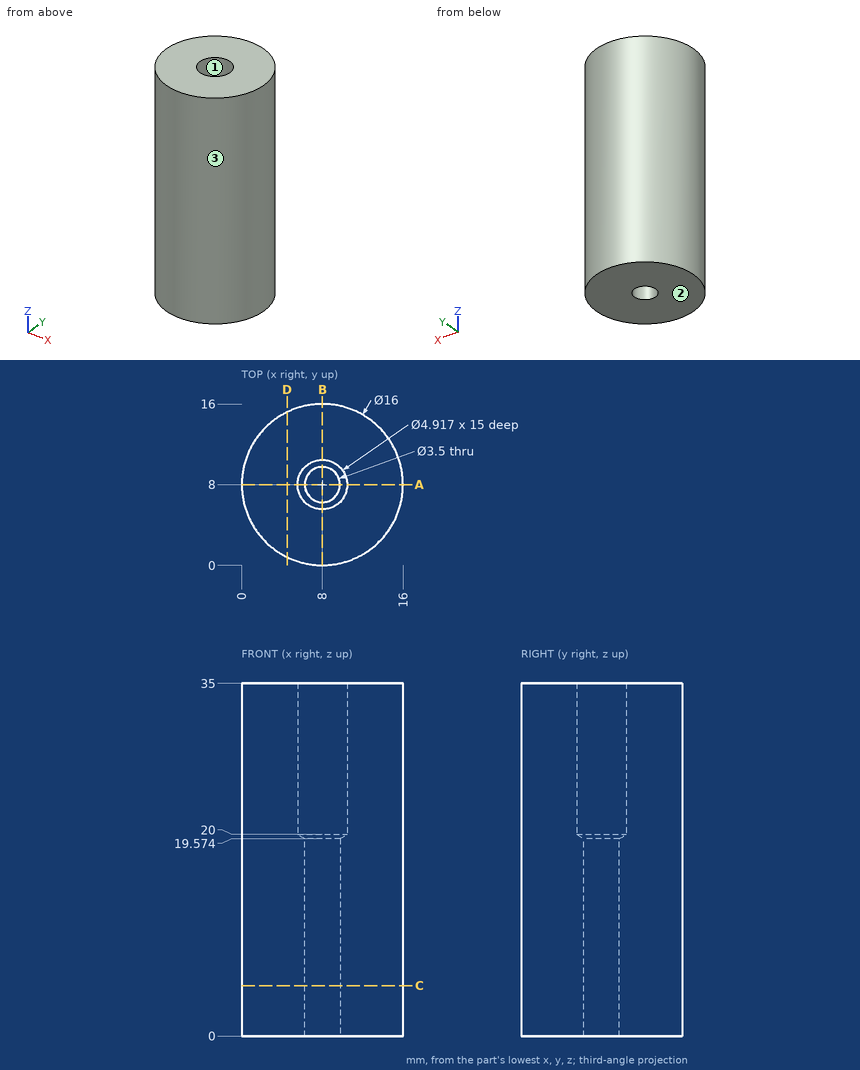
Check sheet for the drawn part. Datum: minimum x, y, z corner. Units: mm. Round coordinates to 2 decimals unless told otherwise and drop trailing zeros. Order: outer loops, then holes, each group sorted by start corner. A loop starts at its lowest first (then second) coordinate and runs counter-clockwise, first axis right, second up. Notation, with made-up numbers: (-24.75, 57) -> (-7.75, 57) arc R18 cw to (-7.75, 90) -> close; hole circle Ø10 at (54, 36). An arc over 180 degrees is marked (long way). Use CSV: the item, a comma, the result in double quotes.
(1) Draft check along Y on the marked faces 1, 2 and 3. Enter one of: pulls with the +Y half, pulls with the -Y half, needs draft (parallel to the pull), parting line crosses it, or undercut.
Worked out:
face 1,"undercut"
face 2,"needs draft"
face 3,"parting line crosses it"
(2) Depth check by flat-ended pin: pin 1 (1.5 mm diameter, centred on y = 4.5, z = 12.5, fed in from +X); pin 2 (2 mm diameter, centred on y = 6.5, z = 29.5, fed in from -X); pin 3 (1 mm diameter, centred on x = 10.5, z = 20.5, fed in from +Y). Enter the tip coordinate at first touch or a pass-through.
Worked out:
pin 1,"x = 15.51"
pin 2,"x = 0.02"
pin 3,"y = 15.75"
(3) Cross-section at C-C (z = 5). Record the boundary of the cut face in (x, y), and give its area (3 significant figures).
Worked out:
outline,"circle Ø16 at (8, 8); hole circle Ø3.5 at (8, 8)"
area,"191 mm²"
(4) Cross-section at A-A (y = 8). Record the boundary of the cut face in (x, z).
Worked out:
outline,"(0, 0) -> (6.25, 0) -> (6.25, 19.57) -> (5.54, 20) -> (5.54, 35) -> (0, 35) -> close; (9.75, 0) -> (16, 0) -> (16, 35) -> (10.46, 35) -> (10.46, 20) -> (9.75, 19.57) -> close"
(5) Cross-section at D-D (x = 4.5). Record the boundary of the cut face in (y, z).
Worked out:
outline,"(0.81, 0) -> (15.19, 0) -> (15.19, 35) -> (0.81, 35) -> close"
(6) Material ranges on line 1 along Y through (x, z) = (8, 12.75); line 2 along X through (y, z) = (7.5, 24.5) (1 decimal); line 3 along X through (y, z) = (6.75, 25), recorded low to high. Write a range as from..to.
Worked out:
line 1,"0..6.25, 9.75..16"
line 2,"0..5.6, 10.4..16"
line 3,"0.1..5.88, 10.12..15.9"
